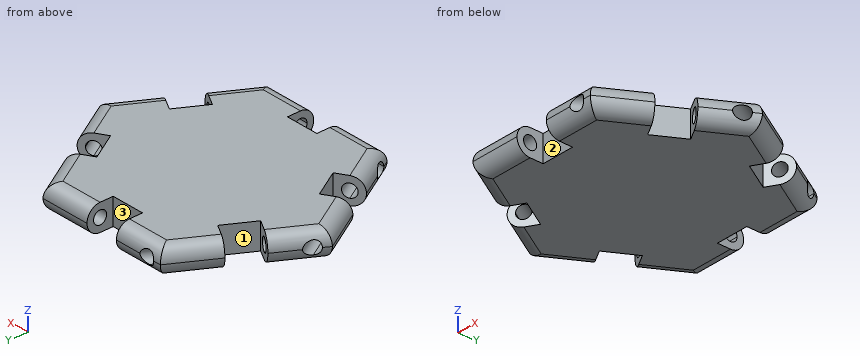
from build123d import *
from build123d import SkipClean  # not in build123d's __all__

# Parameters (mm, degrees)
F1_DEPTH       = 4
F2_W           = 5
F2_H           = 4
F3_DEPTH       = 25
F5_DEPTH       = 3.5
F5_DEPTH_BACK  = 25
F7_DEPTH       = 25
F7_DEPTH_BACK  = 3.5
F9_DEPTH       = 3.5
F9_DEPTH_BACK  = 25
F11_DEPTH      = 25
F11_DEPTH_BACK = 3.5
F13_DEPTH      = 25
F13_DEPTH_BACK = 3.5
F15_DEPTH      = 25
F15_DEPTH_BACK = 3.5
F16_R          = 0.99999
F18_DEPTH      = 25
F18_DEPTH_BACK = 25
F19_DEPTH      = 25
F19_DEPTH_BACK = 25
F20_DEPTH      = 25
F20_DEPTH_BACK = 25
F21_DEPTH      = 25
F21_DEPTH_BACK = 25
F22_DEPTH      = 25
F22_DEPTH_BACK = 25
F23_DEPTH      = 25
F23_DEPTH_BACK = 25


# Not quite as in the source:
# - a fillet or chamfer is up to 0.001 mm smaller than in the source, because OpenCascade refuses the exact size
# - after a boolean that leaves OpenCascade's solid faulty, fix() repairs it


with BuildPart() as f1:
    # F0 (on Top) → F1 (new body)
    with BuildSketch(Plane.XY):
        Polygon((-20, 0), (-10, -17.3205080757), (10, -17.3205080757), (20, 0), (10, 17.3205080757), (-10, 17.3205080757), align=None)
    extrude(amount=F1_DEPTH)

    # F2 (on face) → F3 (cut)
    with BuildSketch(Plane.XY.offset(4)):
        with Locations((0, 15.3205080757)):
            Rectangle(F2_W, F2_H)
        Polygon((12.7858983849, 4.4951905284), (16.25, 6.4951905284), (13.75, 10.8253175473), (10.2858983849, 8.8253175473), align=None)
        Polygon((10.2858983849, -8.8253175473), (13.75, -10.8253175473), (16.25, -6.4951905284), (12.7858983849, -4.4951905284), align=None)
        with Locations((0, -15.3205080757)):
            Rectangle(F2_W, F2_H)
        Polygon((-16.25, -6.4951905284), (-13.75, -10.8253175473), (-10.2858983849, -8.8253175473), (-12.7858983849, -4.4951905284), align=None)
        Polygon((-13.75, 10.8253175473), (-16.25, 6.4951905284), (-12.7858983849, 4.4951905284), (-10.2858983849, 8.8253175473), align=None)
    extrude(amount=-F3_DEPTH, mode=Mode.SUBTRACT)

    # F4 (on face) → F5 (cut, two sides)
    with BuildSketch(Plane(origin=(-1.25, 2.1650635095, 0), x_dir=(0.8660254038, 0.5, 0), z_dir=(0.5, -0.8660254038, 0))) as f5_sk:
        with BuildLine():
            ThreePointArc((16.3205080757, 2), (14.6134012945, 2.7071067812), (15.3205080757, 1))
            ThreePointArc((15.3205080757, 1), (16.0276148569, 1.2928932188), (16.3205080757, 2))
        make_face()
    extrude(amount=-F5_DEPTH, mode=Mode.SUBTRACT)
    extrude(f5_sk.sketch, amount=F5_DEPTH_BACK, mode=Mode.SUBTRACT)

    # F6 (on face) → F7 (cut, two sides)
    with BuildSketch(Plane(origin=(1.25, 2.1650635095, 0), x_dir=(0.8660254038, -0.5, 0), z_dir=(-0.5, -0.8660254038, 0))) as f7_sk:
        with BuildLine():
            ThreePointArc((16.3205080757, 2), (14.6134012945, 2.7071067812), (15.3205080757, 1))
            ThreePointArc((15.3205080757, 1), (16.0276148569, 1.2928932188), (16.3205080757, 2))
        make_face()
    extrude(amount=F7_DEPTH, mode=Mode.SUBTRACT)
    extrude(f7_sk.sketch, amount=-F7_DEPTH_BACK, mode=Mode.SUBTRACT)

    # F8 (on face) → F9 (cut, two sides)
    with BuildSketch(Plane(origin=(2.5, 0, 0), x_dir=(0, -1, 0), z_dir=(-1, 0, 0))) as f9_sk:
        with BuildLine():
            ThreePointArc((16.3205080757, 2), (14.6134012945, 2.7071067812), (15.3205080757, 1))
            ThreePointArc((15.3205080757, 1), (16.0276148569, 1.2928932188), (16.3205080757, 2))
        make_face()
    extrude(amount=-F9_DEPTH, mode=Mode.SUBTRACT)
    extrude(f9_sk.sketch, amount=F9_DEPTH_BACK, mode=Mode.SUBTRACT)

    # F10 (on face) → F11 (cut, two sides)
    with BuildSketch(Plane(origin=(1.25, -2.1650635095, 0), x_dir=(-0.8660254038, -0.5, 0), z_dir=(-0.5, 0.8660254038, 0))) as f11_sk:
        with BuildLine():
            ThreePointArc((16.3205080757, 2), (14.6134012945, 2.7071067812), (15.3205080757, 1))
            ThreePointArc((15.3205080757, 1), (16.0276148569, 1.2928932188), (16.3205080757, 2))
        make_face()
    extrude(amount=F11_DEPTH, mode=Mode.SUBTRACT)
    extrude(f11_sk.sketch, amount=-F11_DEPTH_BACK, mode=Mode.SUBTRACT)

    # F12 (on face) → F13 (cut, two sides)
    with BuildSketch(Plane(origin=(-1.25, -2.1650635095, 0), x_dir=(-0.8660254038, 0.5, 0), z_dir=(0.5, 0.8660254038, 0))) as f13_sk:
        with BuildLine():
            ThreePointArc((16.3205080757, 2), (14.6134012945, 2.7071067812), (15.3205080757, 1))
            ThreePointArc((15.3205080757, 1), (16.0276148569, 1.2928932188), (16.3205080757, 2))
        make_face()
    extrude(amount=F13_DEPTH, mode=Mode.SUBTRACT)
    extrude(f13_sk.sketch, amount=-F13_DEPTH_BACK, mode=Mode.SUBTRACT)

    # F14 (on face) → F15 (cut, two sides)
    with BuildSketch(Plane.YZ.offset(-2.5)) as f15_sk:
        with BuildLine():
            ThreePointArc((16.3205080757, 2), (16.0276148569, 2.7071067812), (15.3205080757, 3))
            ThreePointArc((15.3205080757, 3), (14.6134012945, 1.2928932188), (16.3205080757, 2))
        make_face()
    extrude(amount=F15_DEPTH, mode=Mode.SUBTRACT)
    extrude(f15_sk.sketch, amount=-F15_DEPTH_BACK, mode=Mode.SUBTRACT)

    # F16 (radius 1 in the source; OpenCascade refuses exactly that, so slightly less here)
    f16_edges = [f1.edges().sort_by_distance(p)[0] for p in [
        (-6.25, -17.320508, 4),
        (-6.25, -17.320508, 0),
        (6.25, -17.320508, 4),
        (6.25, -17.320508, 0),
        (11.875, -14.072913, 4),
        (11.875, -14.072913, 0),
        (18.125, -3.247595, 4),
        (18.125, -3.247595, 0),
        (18.125, 3.247595, 4),
        (18.125, 3.247595, 0),
        (11.875, 14.072913, 4),
        (11.875, 14.072913, 0),
        (6.25, 17.320508, 4),
        (6.25, 17.320508, 0),
        (-6.25, 17.320508, 0),
        (-6.25, 17.320508, 4),
        (-11.875, 14.072913, 4),
        (-11.875, 14.072913, 0),
        (-18.125, 3.247595, 4),
        (-18.125, 3.247595, 0),
        (-18.125, -3.247595, 0),
        (-18.125, -3.247595, 4),
        (-11.875, -14.072913, 0),
        (-11.875, -14.072913, 4),
    ]]
    fillet(f16_edges, radius=F16_R)

    # F17 (on face) → F18 (cut, two sides)
    with BuildSketch(Plane(origin=(1.25, -2.1650635095, 0), x_dir=(-0.8660254038, -0.5, 0), z_dir=(-0.5, 0.8660254038, 0))) as f18_sk:
        with BuildLine():
            ThreePointArc((15.3205080757, 4), (16.7347216381, 3.4142135624), (17.3205080757, 2))
            Line((17.3205080757, 2), (17.3205080757, 3.00001))
            ThreePointArc((17.3205080757, 3.00001), (17.0276177858, 3.7071097101), (16.3205180757, 4))
            Line((16.3205180757, 4), (15.3205080757, 4))
        make_face()
        with BuildLine():
            Line((17.3205080757, 0.99999), (17.3205080757, 2))
            ThreePointArc((17.3205080757, 2), (16.7347216381, 0.5857864376), (15.3205080757, 0))
            Line((15.3205080757, 0), (16.3205180757, 0))
            ThreePointArc((16.3205180757, 0), (17.0276177858, 0.2928902899), (17.3205080757, 0.99999))
        make_face()
    extrude(amount=-F18_DEPTH, mode=Mode.SUBTRACT)
    extrude(f18_sk.sketch, amount=F18_DEPTH_BACK, mode=Mode.SUBTRACT)

    # F12 (on face) → F19 (cut, two sides)
    with BuildSketch(Plane(origin=(-1.25, -2.1650635095, 0), x_dir=(-0.8660254038, 0.5, 0), z_dir=(0.5, 0.8660254038, 0))) as f19_sk:
        with BuildLine():
            ThreePointArc((15.3205080757, 4), (16.7347216381, 3.4142135624), (17.3205080757, 2))
            Line((17.3205080757, 2), (17.3205080757, 4))
            Line((17.3205080757, 4), (15.3205080757, 4))
        make_face()
        with BuildLine():
            Line((15.3205080757, 0), (17.3205080757, 0))
            Line((17.3205080757, 0), (17.3205080757, 2))
            ThreePointArc((17.3205080757, 2), (16.7347216381, 0.5857864376), (15.3205080757, 0))
        make_face()
    extrude(amount=-F19_DEPTH, mode=Mode.SUBTRACT)
    extrude(f19_sk.sketch, amount=F19_DEPTH_BACK, mode=Mode.SUBTRACT)

    # F14 (on face) → F20 (cut, two sides)
    with BuildSketch(Plane.YZ.offset(-2.5)) as f20_sk:
        with BuildLine():
            Line((17.3205080757, 2), (17.3205080757, 4))
            Line((17.3205080757, 4), (15.3205080757, 4))
            ThreePointArc((15.3205080757, 4), (16.7347216381, 3.4142135624), (17.3205080757, 2))
        make_face()
        with BuildLine():
            Line((17.3205080757, 0), (17.3205080757, 2))
            ThreePointArc((17.3205080757, 2), (16.7347216381, 0.5857864376), (15.3205080757, 0))
            Line((15.3205080757, 0), (17.3205080757, 0))
        make_face()
    extrude(amount=-F20_DEPTH, mode=Mode.SUBTRACT)
    extrude(f20_sk.sketch, amount=F20_DEPTH_BACK, mode=Mode.SUBTRACT)

    # F6 (on face) → F21 (cut, two sides)
    with BuildSketch(Plane(origin=(1.25, 2.1650635095, 0), x_dir=(0.8660254038, -0.5, 0), z_dir=(-0.5, -0.8660254038, 0))) as f21_sk:
        with BuildLine():
            ThreePointArc((15.3205080757, 4), (16.7347216381, 3.4142135624), (17.3205080757, 2))
            Line((17.3205080757, 2), (17.3205080757, 4))
            Line((17.3205080757, 4), (15.3205080757, 4))
        make_face()
        with BuildLine():
            Line((16.3205080757, 0), (17.3205080757, 0))
            Line((17.3205080757, 0), (17.3205080757, 2))
            ThreePointArc((17.3205080757, 2), (16.7347216381, 0.5857864376), (15.3205080757, 0))
            Line((15.3205080757, 0), (16.3205080757, 0))
        make_face()
    with SkipClean():  # cleaning this boolean's faces spoils the solid; the shape is the same uncleaned
        extrude(amount=-F21_DEPTH, mode=Mode.SUBTRACT)
        extrude(f21_sk.sketch, amount=F21_DEPTH_BACK, mode=Mode.SUBTRACT)

    # F8 (on face) → F22 (cut, two sides)
    with BuildSketch(Plane(origin=(2.5, 0, 0), x_dir=(0, -1, 0), z_dir=(-1, 0, 0))) as f22_sk:
        with BuildLine():
            ThreePointArc((15.3205080757, 4), (16.7347216381, 3.4142135624), (17.3205080757, 2))
            Line((17.3205080757, 2), (17.3205080757, 4))
            Line((17.3205080757, 4), (15.3205080757, 4))
        make_face()
        with BuildLine():
            Line((15.3205080757, 0), (17.3205080757, 0))
            Line((17.3205080757, 0), (17.3205080757, 2))
            ThreePointArc((17.3205080757, 2), (16.7347216381, 0.5857864376), (15.3205080757, 0))
        make_face()
    extrude(amount=-F22_DEPTH, mode=Mode.SUBTRACT)
    extrude(f22_sk.sketch, amount=F22_DEPTH_BACK, mode=Mode.SUBTRACT)

    add(f1.part.fix(), mode=Mode.REPLACE)

    # F4 (on face) → F23 (cut, two sides)
    with BuildSketch(Plane(origin=(-1.25, 2.1650635095, 0), x_dir=(0.8660254038, 0.5, 0), z_dir=(0.5, -0.8660254038, 0))) as f23_sk:
        with BuildLine():
            ThreePointArc((15.3205080757, 4), (16.7347216381, 3.4142135624), (17.3205080757, 2))
            Line((17.3205080757, 2), (17.3205080757, 4))
            Line((17.3205080757, 4), (15.3205080757, 4))
        make_face()
        with BuildLine():
            Line((16.3205080757, 0), (17.3205080757, 0))
            Line((17.3205080757, 0), (17.3205080757, 2))
            ThreePointArc((17.3205080757, 2), (16.7347216381, 0.5857864376), (15.3205080757, 0))
            Line((15.3205080757, 0), (16.3205080757, 0))
        make_face()
    extrude(amount=-F23_DEPTH, mode=Mode.SUBTRACT)
    extrude(f23_sk.sketch, amount=F23_DEPTH_BACK, mode=Mode.SUBTRACT)


solid = f1.part
Input: part model. Units: mm. Frame: model coordinates. Face numbers are marked on the shaded views. A direction names the side the tool comes from. Coordinates: 2 decimals unless noted, no trailing zeros. Loops run counter-clockwise (first coordinate to the right, second up) from the corner with the lowest first, then second, coordinate; pieces in that order, holes last.
(1) Section B-B on y = 5. Count the separate pieces of the cut face and the enclosed holes in it, then the cut area to 3 significant figures.
(2) Set-up query: the marked faces 1, 2 and 3. Return all of +Z, -Z, +X, -X, +Y, -Y with unobstructed straight access to the full face (end or side cutting, diameter ignored); none if empty.
(3) First-contact query: pin 1 Ø2 at (y, z) = (15.5, 1.5) entering from +X; pin 2 Ø1.6 at (y, z) = (-15.32, 2) entering from +X; pin 3 Ø1.5 at (y, z) = (-10, 2.5) entering from -X. Flat tips, straight axial feed; report the tip coordinate or a pass-through.
(4) Material intervals for probe 1 along Y at (x, z) = (5.75, 2); probe 2 along Y at (x, z) = (12.5, 3.45); probe 3 along X at (y, z) = (-4, 2.3), sorted ascending.
(5) Section A-A on x = -4.5. Return the cut outline in (y, z).
Data:
1. separate pieces: 3
1. enclosed holes: 0
1. area: 116 mm2
2. face 1: +Z, -Z
2. face 2: +Z, -Z, -Y
2. face 3: +Z, -Z, +Y
3. pin 1: stops at x = 11.53
3. pin 2: stops at x = 11.62
3. pin 3: stops at x = -13.62
4. probe 1: y = -17.32 to -16.32, -14.32 to 14.32, 16.32 to 17.32
4. probe 2: y = -11.75 to -10.1, -4.99 to 4.99, 10.1 to 11.75
4. probe 3: x = -17.66 to -16.48, -14.28 to 14.28, 16.48 to 17.66
5. outline: (-15.32, 0) - (15.32, 0) arc R2 ccw to (15.32, 4) - (-15.32, 4) arc R2 ccw to start; hole circle Ø2 at (-15.32, 2); hole circle Ø2 at (15.32, 2)
